```python
from build123d import *

# Parameters (mm, degrees)
BOSS_EXTRUDE1_DEPTH     = 4
M3_CLEARANCE_HOLE1_D    = 3.2
FILLET1_R               = 10
TAP_DRILL_FOR_M8_TAP1_D = 6.8
M3_CLEARANCE_HOLE3_D    = 3.4


with BuildPart() as part:
    # Sketch1 → Boss-Extrude1 (new body)
    with BuildSketch(Plane.XY):
        Polygon((128.627293893, -305.665681156), (128.627293893, -359.464720764), (-108.372706107, -359.464720764), (-108.372706107, -305.665681156), (-108.372706107, -271.718782294), (-72.968170503, -271.718782294), (-72.968170503, -303.597286204), (93.222758289, -303.597286204), (93.222758289, -271.718782294), (128.627293893, -271.718782294), align=None)
    extrude(amount=BOSS_EXTRUDE1_DEPTH)

    # M3 Clearance Hole1 (through all)
    with Locations(Plane.XY.offset(4)):
        with Locations((-82.072706107, -292.415681156), (115.327293893, -292.415681156), (90.417293893, -320.915681156), (-57.162706107, -320.915681156)):
            Hole(M3_CLEARANCE_HOLE1_D / 2)

    # Fillet1
    fillet1_edges = [part.edges().sort_by_distance(p)[0] for p in [
        (128.627293893, -359.464720764, 2),
        (-108.372706107, -359.464720764, 2),
        (-108.372706107, -271.718782294, 2),
        (-72.968170503, -271.718782294, 2),
        (-72.968170503, -303.597286204, 2),
        (93.222758289, -303.597286204, 2),
        (93.222758289, -271.718782294, 2),
        (128.627293893, -271.718782294, 2),
    ]]
    fillet(fillet1_edges, radius=FILLET1_R)

    # Tap Drill for M8 Tap1 (through all)
    with Locations(Plane.XY.offset(4)):
        with Locations((78.681014792, -344.935502047), (-45.318985208, -344.935502047)):
            Hole(TAP_DRILL_FOR_M8_TAP1_D / 2)

    # M3 Clearance Hole3 (through all)
    with Locations(Plane.XY.offset(4)):
        with Locations((52.592509681, -330.665681156), (52.592509681, -357.226830961), (-57.162706107, -357.226830961)):
            Hole(M3_CLEARANCE_HOLE3_D / 2)


solid = part.part
```
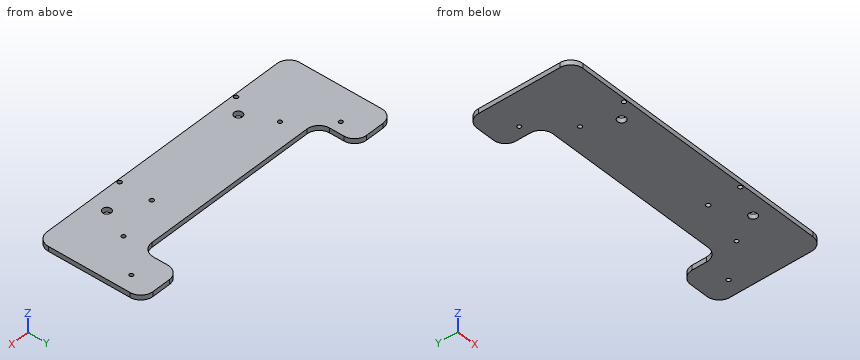
Input: part model. Units: mm. Frame: model coordinates. Give positions to 0.01 mm unless a question says otherwise; leave off trailing zeros. Order: outer loops, then holes, each group sorted by start corner. A loop starts at its lowest first (then second) coordinate and runs counter-clockwise, first axis right, second up. Notation, with made-up numbers: (10, 1.5) - (36, 1.5) arc R30 cw to (36, 33.5) - close; hole circle Ø3 at (30.5, -20). An arc over 180 degrees is marked (long way). One line per item, written item: value.
1. Cut plane C-C, the plane x = 7. Output: boundary loops of the cut face in (y, z).
Determined:
outline: (-359.46, 0) - (-303.6, 0) - (-303.6, 4) - (-359.46, 4) - close
2. Pin query (flat end, axial travel): pin 1 Ø3 at (x, y) = (-82.07, -292.42) entering from +Z; pin 2 Ø1.5 at (x, z) = (14.5, 1.5) entering from +Y. Return the tip coordinate at first contact, or that it passes through.
Determined:
pin 1: through
pin 2: y = -303.6
3. Cut plane A-A, the plane y = -288. Output: boundary loops of the cut face in (x, z).
Determined:
outline: (-108.37, 0) - (-72.97, 0) - (-72.97, 4) - (-108.37, 4) - close; (93.22, 0) - (128.63, 0) - (128.63, 4) - (93.22, 4) - close
4. Cut plane D-D, the plane x = 98. Output: boundary loops of the cut face in (y, z).
Determined:
outline: (-359.46, 0) - (-273.19, 0) - (-273.19, 4) - (-359.46, 4) - close
5. Cut plane B-B, the plane z = 1.8. Give the number of separate pieces and of enclosed holes in the cut face, and give its area (3 significant figures).
Determined:
separate pieces: 1
enclosed holes: 9
area: 15,300 mm2
6. Line query: probe 1 along X at (y, z) = (-321, 2.75); probe 2 along Y at (x, z) = (-45.5, 0.6); probe 3 along X at (y, z) = (-320, 0.45). Output: solid intervals per line, ascending.
Determined:
probe 1: -108.37 to -58.76, -55.56 to 88.82, 92.02 to 128.63
probe 2: -359.46 to -348.33, -341.54 to -303.6
probe 3: -108.37 to -58.47, -55.85 to 89.11, 91.73 to 128.63
